Model file for the job. Use its own axes, mm. A direction names the side the tool comes from. Round coordinates to 2 decimals unless told otherwise and drop trailing zeros. Loops run counter-clockwise (first coordinate to the right, second up) from the corner with the lowest first, then second, coordinate; pieces in that order, holes last. Notation, with made-up numbers: (-4, 34) - (4, 34) arc R24 ccw to (4, 45) - close; hole circle Ø4 at (-32.75, -33). An arc over 180 degrees is marked (long way). Answer as a JSON object with one key per item and string values.
from build123d import *

# Parameters (mm, degrees)
SKETCH014_W             = 100
SKETCH014_H             = 300
PAD012_DEPTH            = 5
SKETCH037_W             = 10
SKETCH037_H             = 5
POCKET008_DEPTH         = 5
LINEARPATTERN017_COUNT  = 5
LINEARPATTERN017_PITCH  = 20
SKETCH038_W             = 10
SKETCH038_H             = 5
POCKET009_DEPTH         = 5
LINEARPATTERN018_COUNT  = 5
LINEARPATTERN018_PITCH  = 20
SKETCH039_W             = 10
SKETCH039_H             = 5
POCKET010_DEPTH         = 5
LINEARPATTERN019_COUNT  = 15
LINEARPATTERN019_PITCH  = 20
BODY012_PLACEMENT_ANGLE = 90


with BuildPart() as part:
    # Sketch014 → Pad012 (new body)
    with BuildSketch(Plane.XY):
        Rectangle(SKETCH014_W, SKETCH014_H)
    extrude(amount=PAD012_DEPTH)

    # Sketch037 (on DatumPlane) → Pocket008 (cut)
    with BuildSketch(Plane.XZ.offset(150)):
        with Locations((-40, 2.5)):
            Rectangle(SKETCH037_W, SKETCH037_H)
    pocket008 = extrude(amount=-POCKET008_DEPTH, mode=Mode.SUBTRACT)

    # LinearPattern017: Pocket008 ×5
    with Locations(*[(i * LINEARPATTERN017_PITCH, 0, 0) for i in range(1, LINEARPATTERN017_COUNT)]):
        add(pocket008, mode=Mode.SUBTRACT)

    # Sketch038 (on DatumPlane) → Pocket009 (cut)
    with BuildSketch(Plane(origin=(0, 150, 0), x_dir=(-1, 0, 0), z_dir=(0, 1, 0))):
        with Locations((-40, 2.5)):
            Rectangle(SKETCH038_W, SKETCH038_H)
    pocket009 = extrude(amount=-POCKET009_DEPTH, mode=Mode.SUBTRACT)

    # LinearPattern018: Pocket009 ×5
    with Locations(*[(-i * LINEARPATTERN018_PITCH, 0, 0) for i in range(1, LINEARPATTERN018_COUNT)]):
        add(pocket009, mode=Mode.SUBTRACT)

    # Sketch039 (on DatumPlane) → Pocket010 (cut)
    with BuildSketch(Plane.YZ.offset(50)):
        with Locations((-135, 2.5)):
            Rectangle(SKETCH039_W, SKETCH039_H)
    pocket010 = extrude(amount=-POCKET010_DEPTH, mode=Mode.SUBTRACT)

    # LinearPattern019: Pocket010 ×15
    with Locations(*[(0, i * LINEARPATTERN019_PITCH, 0) for i in range(1, LINEARPATTERN019_COUNT)]):
        add(pocket010, mode=Mode.SUBTRACT)


with BuildPart() as part_1:
    # Body012 placement: moved
    add(part.part.moved(Location((-250, 0, 155))).rotate(Axis((-250, 0, 155), (0, -1, 0)), BODY012_PLACEMENT_ANGLE))


solid = part_1.part
1) Two-plate mould, pull along Y, no slides. Class faces 1 (the flat face through (-252, 90, 203)), 2 (the flat face through (-252, 10, 203)), 3 (the flat face through (-253, -145, 175)), 4 (the flat face through (-252, 55, 205)): pulls with the +Y half, pulls with the -Y half, needs draft (parallel to the pull), parting line crosses it, or undercut.
Values follow:
{"face 1": "undercut", "face 2": "undercut", "face 3": "pulls with the -Y half", "face 4": "needs draft"}
2) Slice it at B-B on y = -35.5. List the corners of the cut face in (x, z).
Values follow:
{"outline": "(-255, 105) - (-250, 105) - (-250, 200) - (-255, 200) - close"}
3) Drop flat-ended pins along their axis: P1, Ø2.5, axis at x = -251.5, z = 133, coming from the -Y side; P2, Ø2.5, axis at x = -252, y = 2.5, coming from the +Z side; P3, Ø1.5, axis at x = -253, z = 202, coming from the +Y side. Give the stop position or say it passes through.
Values follow:
{"P1": "y = -145", "P2": "z = 200", "P3": "y = 140"}
4) Slice it at A-A on z = 153.5. List the corners of the cut face in (x, y), then the cut area to 3 significant figures.
Values follow:
{"outline": "(-255, -145) - (-250, -145) - (-250, 145) - (-255, 145) - close", "area": "1,450 mm²"}
5) Tool access for faces 5 (the flat face through (-253, 142, 200)), 6 (the flat face through (-252, -10, 203)), 7 (the flat face through (-252, -148, 130)), 8 (the flat face through (-252, 148, 120)): list every direction of +Z, -Z, +X, -X, +Y, -Y with a clear straight run to the whole face (end or side of a thin tool).
Values follow:
{"face 5": "+Z, +X, -X, +Y", "face 6": "+Z, +X, -X", "face 7": "+X, -X, -Y", "face 8": "+X, -X, +Y"}
6) Probe probe 1 along Z at (x, y) = (-252.3, -39); probe 2 along Y at (x, z) = (-250.55, 150.5). List the from-to ranges inside material, lowest first.
Values follow:
{"probe 1": "105 to 200", "probe 2": "-145 to 145"}
